Can you work these out from the drawing? Everything is in mm from the part's minimum corner. Coordinates: 2 decimals unless noted, no trailing zeros. Order: outer loops, then holes, each group sorted by start corner. A loop starts at its lowest first (then second) coordinate and runs counter-clockwise, first axis right, second up. Notation, with made-up numbers: (53, -34.75) -> (60, -34.75) arc R30 cw to (60, -4.75) -> close; hole circle Ø10 at (38, 7.5). An arc over 180 degrees is marked (long way). Return JSON: item names as keys, results as strings. Group by question number.
1) If we section it at D-D, the plane y = 4.15: Please give me the cut outline in (x, z).
2) If we section it at C-C, the plane z = 6: Please give me the cut outline in (x, y).
3) If we section it at A-A, the plane x = 2.25: Please give me the cut outline in (y, z), then the cut area to 3 significant figures.
4) Thinking about a two-plate mould opening in Z: for the marked faces 1, 2 and 3, which applies, +Z half, -Z half, draft (parallel to the pull), parting line (faces both ways), or undercut?
5) If I drill on probe 1 along Z at (x, y) = (3.8, 3.3); probe 2 along Y at (x, z) = (2.3, 2.5); probe 3 along X at (y, z) = (0.95, 5), over which ranges is the centre line in solid material (lowest first)? Write a range as from..to.
6) For pin 1 (1 mm diameter, centred on y = 2, z = 10.5, fed in from -X); pin 2 (1.5 mm diameter, centred on x = 1.5, z = 9.5, fed in from -Y); pin 3 (1 mm diameter, centred on y = 1, z = 5.5, fed in from +X), each with a flat end and sliding along its axis, tell me the tip position at first contact or that it passes through.
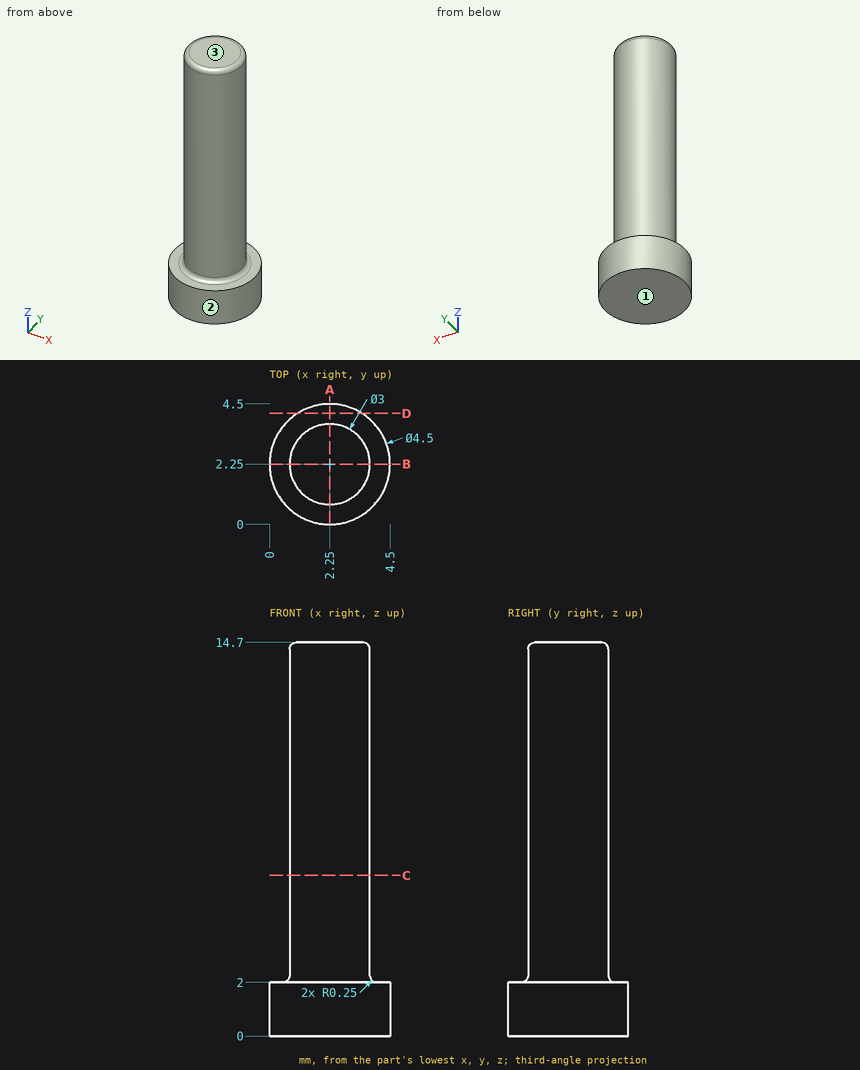
Result sheet:
{
 "1": {"outline": "(1.04, 0) -> (3.46, 0) -> (3.46, 2) -> (1.04, 2) -> close"},
 "2": {"outline": "circle Ø3 at (2.25, 2.25)"},
 "3": {"outline": "(0, 0) -> (4.5, 0) -> (4.5, 2) -> (4, 2) arc R0.25 cw to (3.75, 2.25) -> (3.75, 14.45) arc R0.25 ccw to (3.5, 14.7) -> (1, 14.7) arc R0.25 ccw to (0.75, 14.45) -> (0.75, 2.25) arc R0.25 cw to (0.5, 2) -> (0, 2) -> close", "area": "47.1 mm2"},
 "4": {"face 1": "-Z half", "face 2": "draft", "face 3": "+Z half"},
 "5": {"probe 1": "z = 0..2", "probe 2": "y = 0.75..3.75", "probe 3": "x = 1.5..3"},
 "6": {"pin 1": "stops at x = 0.75", "pin 2": "stops at y = 0.75", "pin 3": "stops at x = 3.55"}
}
